```python
from build123d import *


with BuildPart() as part:
    # Austragung1: sweep along a path in Skizze1
    with BuildLine(Plane(origin=(0, 0, 0), x_dir=(1, 0, 0), z_dir=(0, 1, 0))) as austragung1_path:
        Line((-100.35104183, -57.432811357), (100.35104183, -57.432811357))
        ThreePointArc((100.35104183, -57.432811357), (114.493177454, -51.574946981), (120.35104183, -37.432811357))
        Line((120.35104183, -37.432811357), (120.35104183, 37.432811357))
        ThreePointArc((120.35104183, 37.432811357), (114.493177454, 51.574946981), (100.35104183, 57.432811357))
        Line((100.35104183, 57.432811357), (-100.35104183, 57.432811357))
        ThreePointArc((-100.35104183, 57.432811357), (-110.666950496, 54.567046922), (-118.026562745, 46.791014197))
        ThreePointArc((-118.026562745, 46.791014197), (-129.64895817, 0), (-118.026562745, -46.791014197))
        ThreePointArc((-118.026562745, -46.791014197), (-110.666950496, -54.567046922), (-100.35104183, -57.432811357))
    # Skizze2 → Austragung1 (sweep)
    with BuildSketch(Plane.XY):
        with BuildLine():
            Line((-124.64895817, 0), (-124.64895817, -15))
            ThreePointArc((-124.64895817, -15), (-129.64895817, -20), (-134.64895817, -15))
            Line((-134.64895817, -15), (-134.64895817, 0))
            ThreePointArc((-134.64895817, 0), (-129.64895817, 5), (-124.64895817, 0))
        make_face()
    sweep(path=austragung1_path.line)


solid = part.part
```
Here's how the part is built. I have some questions about the finished solid (model axes, mm). A direction names the side the tool comes from. Round coordinates to 2 decimals unless told otherwise and drop trailing zeros. Loops run counter-clockwise (first coordinate to the right, second up) from the corner with the lowest first, then second, coordinate; pieces in that order, holes last.
1. Will these pins go through, and if not, where does the flat tip stop? pin 1 (8 mm diameter, centred on y = -12, z = -19.5, fed in from -X); pin 2 (4.5 mm diameter, centred on y = -8.5, z = -18, fed in from -X); pin 3 (6 mm diameter, centred on y = -13.5, z = -7, fed in from -X).
Answers:
pin 1: stops at x = -133.5
pin 2: stops at x = -133.46
pin 3: stops at x = -134.57
2. If I drill on probe 1 along Z at (x, y) = (95, -5.5); probe 2 along Z at (x, y) = (21.5, -15.5); probe 3 along X at (y, z) = (-11.5, -40.5), over which ranges is the centre line in solid material (lowest first)?
Answers:
probe 1: z = -62.43 to -52.43, 52.43 to 62.43
probe 2: z = -62.41 to -52.46, 52.46 to 62.41
probe 3: x = -126.52 to -115.58, 115.03 to 125.16
3. Suppose I cut it at C-C, the plane z = 0. Please give me the cut outline in (x, y), and give its area (3 significant figures).
Answers:
outline: (-134.65, -15) arc R5 ccw to (-124.65, -15) - (-124.65, 0) arc R5 ccw to (-134.65, 0) - close; (115.35, -15) arc R5 ccw to (125.35, -15) - (125.35, 0) arc R5 ccw to (115.35, 0) - close
area: 457 mm2
4. Suppose I cut it at B-B, the plane y = -8. Please give me the cut outline in (x, z), and give its area (3 significant figures).
Answers:
outline: (-122.45, -49.13) arc R25 ccw to (-100.35, -62.43) - (100.35, -62.43) arc R25 ccw to (125.35, -37.43) - (125.35, 37.43) arc R25 ccw to (100.35, 62.43) - (-100.35, 62.43) arc R25 ccw to (-122.45, 49.13) arc R105 ccw to start; hole (-113.61, -44.45) arc R15 ccw to (-100.35, -52.43) - (100.35, -52.43) arc R15 ccw to (115.35, -37.43) - (115.35, 37.43) arc R15 ccw to (100.35, 52.43) - (-100.35, 52.43) arc R15 ccw to (-113.61, 44.45) arc R95 ccw to start
area: 6,800 mm2
5. Thinking about a two-plate mould opening in Z: for faces 4 (the face through (-1.4, -20, -57.5)), 5 (the face through (-113.41, -7.6, 58.75)), 6 (the face through (118.222, -7.605, -54.915)), which applies, released by +Z, released by -Z, zero draft, split by the parting line, or undercut?
Answers:
face 4: undercut
face 5: released by +Z
face 6: released by -Z
6. Suppose I cut it at A-A, the plane x = -11. Please give me the cut outline in (y, z), and give its area (3 significant figures).
Answers:
outline: (-15, -62.43) - (0, -62.43) arc R5 ccw to (0, -52.43) - (-15, -52.43) arc R5 ccw to start; (-15, 52.43) - (0, 52.43) arc R5 ccw to (0, 62.43) - (-15, 62.43) arc R5 ccw to start
area: 457 mm2
7. For faces 1 (the face through (-1, -8, -52.433)), 2 (the face through (1.4, -20, 57.5)), 3 (the face through (1.4, 5, 57.3)), which set-ups out of +Z, -Z, +X, -X, +Y, -Y let a thin tool reach every point of the face, with its end or its side?
Answers:
face 1: +Y, -Y
face 2: -Y
face 3: +Y
